Part model, mm, in its own coordinate system. Face numbers are marked on the shaded views. A direction names the side the tool comes from. Coordinates: 2 decimals unless noted, no trailing zeros. Order: outer loops, then holes, each group sorted by start corner. A loop starts at its lowest first (then second) coordinate and runs counter-clockwise, first axis right, second up.
1) Pin check, flat tips, straight feed: pin 1 Ø1.5 at (x, y) = (-235, 100) entering from +Z; pin 2 Ø15 at (y, z) = (36.5, -0.5) entering from -X; pin 3 Ø23.5 at (y, z) = (193, -62.5) entering from +X. Stop position of each tip, or through.
2) Cut at D-D (x = -58). List the corners of the cut face in (y, z), and give its area (4 significant figures).
3) Wall check: L1, parallel to Z at x = 58, y = 53.5; L2, parallel to Y at x = 178, z = 92.5; L3, parallel to X at y = 15.5, z = 9. Give the ranges that are in metal, low to high.
4) Mould opens along Z. For the marked faces 1, 2 and 3 say: +Z half, -Z half, draft (parallel to the pull), parting line (faces both ways), or undercut.
5) Cut at B-B (z = 89). List the corners of the cut face in (x, y), and give its area (3 significant figures).
6) Cut at A-A (x = -236). List the corners of the cut face in (y, z), and give its area (3 significant figures).
7) Cut at C-C (z = 11). List the corners of the cut face in (x, y).
8) Tool access for the marked faces 4, 5, 6 and 7: list every direction of +Z, -Z, +X, -X, +Y, -Y with a clear straight run to the whole face (end or side of a thin tool).
```python
from build123d import *

# Parameters (mm, degrees)
BOSS_EXTRUDE1_DEPTH = 350
SKETCH2_W           = 54
SKETCH2_H           = 125
BOSS_EXTRUDE2_DEPTH = 36
SKETCH4_W           = 54
SKETCH4_H           = 125
BOSS_EXTRUDE3_DEPTH = 50
SKETCH5_R           = 15
CUT_EXTRUDE1_DEPTH  = 25
SKETCH6_W           = 70
SKETCH6_H           = 30
BOSS_EXTRUDE4_DEPTH = 10
SKETCH7_W           = 50
SKETCH7_H           = 20
BOSS_EXTRUDE5_DEPTH = 100
BOSS_EXTRUDE6_DEPTH = 75


with BuildPart() as part:
    # Sketch1 → Boss-Extrude1 (new body, symmetric)
    with BuildSketch(Plane(origin=(0, 0, 0), x_dir=(0, 0, -1), z_dir=(1, 0, 0))):
        Polygon((-120, -30), (120, -30), (120, 50), (70, 50), (70, 70), (45, 70), (45, 0), (-80, 0), (-80, 100), (-105, 100), (-105, 50), (-120, 50), align=None)
    extrude(amount=BOSS_EXTRUDE1_DEPTH, both=True)

    # Sketch2 → Boss-Extrude2 (add)
    with BuildSketch(Plane(origin=(0, 0, 0), x_dir=(1, 0, 0), z_dir=(0, 1, 0))):
        with Locations((-323, -17.5)):
            Rectangle(SKETCH2_W, SKETCH2_H)
    extrude(amount=BOSS_EXTRUDE2_DEPTH)

    # Sketch4 → Boss-Extrude3 (add)
    with BuildSketch(Plane(origin=(0, 0, 0), x_dir=(1, 0, 0), z_dir=(0, 1, 0))):
        with Locations((323, -17.5)):
            Rectangle(SKETCH4_W, SKETCH4_H)
    extrude(amount=BOSS_EXTRUDE3_DEPTH)

    # Sketch5 → Cut-Extrude1 (cut)
    with BuildSketch(Plane(origin=(0, 0, 80), x_dir=(-1, 0, 0), z_dir=(0, 0, -1))):
        with Locations((-178, 75)):
            Circle(SKETCH5_R)
        with Locations((-60, 75)):
            Circle(SKETCH5_R)
        with Locations((58, 75)):
            Circle(SKETCH5_R)
    extrude(amount=-CUT_EXTRUDE1_DEPTH, mode=Mode.SUBTRACT)

    # Sketch6 → Boss-Extrude4 (add)
    with BuildSketch(Plane(origin=(0, 50, 0), x_dir=(1, 0, 0), z_dir=(0, 1, 0))):
        with Locations((-285, 95)):
            Rectangle(SKETCH6_W, SKETCH6_H)
    extrude(amount=BOSS_EXTRUDE4_DEPTH)

    # Sketch7 → Boss-Extrude5 (add)
    with BuildSketch(Plane(origin=(0, 60, 0), x_dir=(1, 0, 0), z_dir=(0, 1, 0))):
        with Locations((-285, 95)):
            Rectangle(SKETCH7_W, SKETCH7_H)
    extrude(amount=BOSS_EXTRUDE5_DEPTH)

    # Sketch10 → Boss-Extrude6 (add, symmetric)
    with BuildSketch(Plane.ZY.offset(285)):
        with BuildLine():
            Line((-105, 160), (-85, 160))
            Line((-85, 160), (-35, 246.602540378))
            Line((-35, 246.602540378), (-39.330127019, 249.102540378))
            Line((-39.330127019, 249.102540378), (-86.830127019, 166.830127019))
            ThreePointArc((-86.830127019, 166.830127019), (-89.866158812, 164.500497887), (-93.660254038, 165))
            Line((-93.660254038, 165), (-110.980762114, 175))
            Line((-110.980762114, 175), (-113.480762114, 170.669872981))
            Line((-113.480762114, 170.669872981), (-105, 160))
        make_face()
    extrude(amount=BOSS_EXTRUDE6_DEPTH, both=True)


solid = part.part
```
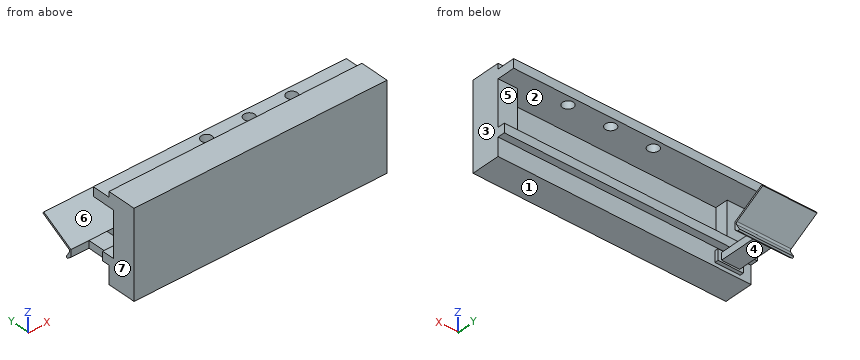
Geometry check:
1. pin 1: stops at z = 105
1. pin 2: stops at x = -350
1. pin 3: stops at x = -210
2. outline: (-30, -120) - (50, -120) - (50, -70) - (70, -70) - (70, -45) - (0, -45) - (0, 80) - (60, 80) - (60, 105) - (50, 105) - (50, 120) - (-30, 120) - close; (90, 80) - (100, 80) - (100, 105) - (90, 105) - close
2. area: 13,950 mm2
3. L1: z = -70 to -45, 80 to 105
3. L2: y = -30 to 60, 90 to 100
3. L3: x = -350 to -296, 296 to 350
4. face 1: -Z half
4. face 2: undercut
4. face 3: draft
5. outline: (-350, -30) - (350, -30) - (350, 100) - (-350, 100) - close; hole circle Ø30 at (-58, 75); hole circle Ø30 at (60, 75); hole circle Ø30 at (178, 75)
5. area: 88,900 mm2
6. outline: (-30, -120) - (50, -120) - (50, -70) - (70, -70) - (70, -45) - (0, -45) - (0, 80) - (100, 80) - (100, 105) - (50, 105) - (50, 120) - (-30, 120) - close; (160, -105) - (170.67, -113.48) - (175, -110.98) - (165, -93.66) arc R5 cw to (166.83, -86.83) - (249.1, -39.33) - (246.6, -35) - (160, -85) - close
6. area: 15,400 mm2
7. outline: (-350, -30) - (350, -30) - (350, 50) - (296, 50) - (296, 0) - (-296, 0) - (-296, 36) - (-350, 36) - close
8. face 4: -Z, +X, -X
8. face 5: +X, -X, +Y
8. face 6: +Z, +X, -X
8. face 7: +Z, -Z, -X, -Y
